from build123d import *

# Parameters (mm, degrees)
SKETCH1_W               = 20
SKETCH1_H               = 10
BOSS_EXTRUDE1_DEPTH     = 6.2
SKETCH2_R               = 0.9
BOSS_EXTRUDE2_DEPTH     = 2
FILLET1_R               = 2
CUT_EXTRUDE1_DEPTH      = 14.86506401
CUT_EXTRUDE1_DEPTH_BACK = 2
SKETCH3_R               = 5.005
CUT_EXTRUDE2_DEPTH      = 13.784365452
CUT_EXTRUDE2_DEPTH_BACK = 13.784365452
CUT_EXTRUDE3_DEPTH      = 5


with BuildPart() as part:
    # Sketch1 → Boss-Extrude1 (new body)
    with BuildSketch(Plane.YZ):
        Rectangle(SKETCH1_W, SKETCH1_H)
    extrude(amount=BOSS_EXTRUDE1_DEPTH)

    # Sketch2 → Boss-Extrude2 (add)
    with BuildSketch(Plane.YZ):
        with Locations(Location((-4.75, 3, 0), (0, 0, 270))):
            Circle(SKETCH2_R)
        with Locations(Location((4.75, 3, 0), (0, 0, 90))):
            Circle(SKETCH2_R)
    extrude(amount=-BOSS_EXTRUDE2_DEPTH)

    # Fillet1
    fillet1_edges = [part.edges().sort_by_distance(p)[0] for p in [
        (3.1, -10, 5),
        (3.1, 10, 5),
    ]]
    fillet(fillet1_edges, radius=FILLET1_R)

    # Sketch3 → Cut-Extrude1 (cut, two sides: drawn at the far end of the back side and taken through both)
    with BuildSketch(Plane.YZ.offset(6.2).offset(-CUT_EXTRUDE1_DEPTH_BACK)):
        Circle(SKETCH3_R)
    extrude(amount=CUT_EXTRUDE1_DEPTH + CUT_EXTRUDE1_DEPTH_BACK, mode=Mode.SUBTRACT)

    # Sketch4 → Cut-Extrude2 (cut, two sides: drawn at the far end of the back side and taken through both)
    with BuildSketch(Plane(origin=(0, 0, 0), x_dir=(-1, 0, 0), z_dir=(0, 1, 0)).offset(-CUT_EXTRUDE2_DEPTH_BACK)):
        with BuildLine():
            Line((-4.2, -5), (0, -5))
            Line((0, -5), (0, 0))
            ThreePointArc((0, 0), (-2.922321699, -1.809249773), (-4.2, -5))
        make_face()
    extrude(amount=CUT_EXTRUDE2_DEPTH + CUT_EXTRUDE2_DEPTH_BACK, mode=Mode.SUBTRACT)

    # Sketch5 → Cut-Extrude3 (cut)
    with BuildSketch(Plane.YZ.offset(6.2)):
        with BuildLine():
            Line((-10, 5), (-2.291287847, 5))
            ThreePointArc((-2.291287847, 5), (-5.5, 0), (-2.291287847, -5))
            Line((-2.291287847, -5), (-10, -5))
            Line((-10, -5), (-10, 5))
        make_face()
        with BuildLine():
            Line((10, 5), (10, -5))
            Line((10, -5), (2.291287847, -5))
            ThreePointArc((2.291287847, -5), (5.5, 0), (2.291287847, 5))
            Line((2.291287847, 5), (10, 5))
        make_face()
    extrude(amount=-CUT_EXTRUDE3_DEPTH, mode=Mode.SUBTRACT)


solid = part.part
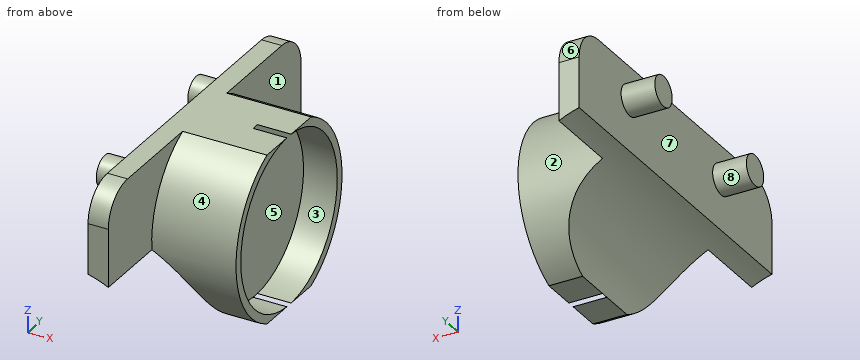
Geometry: final body of the model. Coordinates: model frame, mm. Face numbers are marked on the shaded views. A direction names the side the tool comes from. Give positions to 0.01 mm unless a question says otherwise; leave off trailing zeros. Loops run counter-clockwise (first coordinate to the right, second up) from the corner with the lowest first, then second, coordinate; pieces in that order, holes last. Notation, with made-up numbers: (-39.75, -8.5) - (3.25, -8.5) arc R18 ccw to (3.25, 6.5) - close; hole circle Ø6 at (54, 73). An arc over 180 degrees is marked (long way). Answer as CSV lines item,"result". Start each with the question number.
1. Section A-A, the plane x = 4.5. Return loops of the section in (y, z) (3 decimals), plus the area to 3 significant figures.
2. Section B-B, the plane y = 6.25. Return loops of the section in (x, z).
3. Section D-D, the plane x = 1. Return loops of the section in (y, z), plus the area to 3 significant figures.
4. Section C-C, the plane z = 2.5. Return loops of the section in (x, y), plus the area to 3 significant figures.
5. Ray query, L1, parallel to X at y = -5.75, z = 1; L2, parallel to X at y = -2, z = 3.5; L3, parallel to Y at x = 5.25, z = 1.5. Return the intervals inside material, ascending.
6. Pin query (flat end, axial travel): P1, Ø1, axis at x = 2, y = 6.5, coming from the +Z side; P2, Ø3, axis at y = 0, z = 2.5, coming from the +X side; P3, Ø1.5, axis at x = 2.5, z = 2, coming from the -Y side. Return the tip coordinate at first contact, or that it passes through.
7. Draft query along Z for the marked faces 5, 6, 7 and 8. Return one class per face: released by +Z, released by -Z, zero draft, split by the parting line, or undercut.
8. Reachability of the marked faces 1, 2, 3 and 4 from +Z, -Z, +X, -X, +Y, -Y: full face, straight path, thin tool, end or side. Return the list, or none.
Answers:
1,outline,"(-2.291, -5) - (-0.224, -5) arc R5.005 cw to (-0.224, 5) - (-2.291, 5) arc R5.5 ccw to start; (0.224, -5) - (2.291, -5) arc R5.5 ccw to (2.291, 5) - (0.224, 5) arc R5.005 cw to start"
1,area,"13.3 mm2"
2,outline,"(0, 0) arc R5.5 cw to (1.2, -0.44) - (1.2, 5) - (0, 5) - close"
3,outline,"(-10, -0.35) - (10, -0.35) - (10, 3) arc R2 ccw to (8, 5) - (-8, 5) arc R2 ccw to (-10, 3) - close"
3,area,"105 mm2"
4,outline,"(-2, -5.5) - (0, -5.5) - (0, -10) - (1.2, -10) - (1.2, -4.9) - (6.2, -4.9) - (6.2, -4.34) - (4.2, -4.34) - (4.2, 4.34) - (6.2, 4.34) - (6.2, 4.9) - (1.2, 4.9) - (1.2, 10) - (0, 10) - (0, 5.5) - (-2, 5.5) - (-2, 4) - (0, 4) - (0, -4) - (-2, -4) - close"
4,area,"61.6 mm2"
5,L1,"x = 0 to 1.2"
5,L2,"x = 0 to 4.2"
5,L3,"y = -5.29 to -4.77, 4.77 to 5.29"
6,P1,"passes through"
6,P2,"stops at x = 4.2"
6,P3,"stops at y = -5.36"
7,face 5,"undercut"
7,face 6,"released by +Z"
7,face 7,"zero draft"
7,face 8,"split by the parting line"
8,face 1,"+Z, +X, +Y"
8,face 2,"+X, +Y"
8,face 3,"+X"
8,face 4,"+X, -Y"
